Work out the finished part from the listing and answer in its coordinate system (mm). Face numbers are marked on the shaded views. A direction names the side the tool comes from. Round coordinates to 2 decimals unless told otherwise and drop trailing zeros. Order: outer loops, then holes, each group sorted by start corner. A loop starts at its lowest first (then second) coordinate and runs counter-clockwise, first axis right, second up.
Autodesk Inventor part; units mm, degrees
ref_plane "YZ Plane" through (0, 0, 0) normal (1, 0, 0) x (0, 1, 0)
ref_plane "XZ Plane" through (0, 0, 0) normal (0, 1, 0) x (-1, 0, 0)
ref_plane "XY Plane" through (0, 0, 0) normal (0, 0, 1) x (1, 0, 0)
sketch "Skizze1" plane through (0, 0, 0) normal (0, 1, 0) x (-1, 0, 0)
  line L0 (12.5, 72.5) -> (-12.5, 72.5)
  line L1 (-12.5, 72.5) -> (-12.5, -72.5)
  line L2 (-12.5, -72.5) -> (12.5, -72.5)
  line L3 (12.5, -72.5) -> (12.5, 72.5)
  point P0 (0, 0)
  point P1 (0, 72.5)
  point P2 (-12.5, 0)
  dimension "d0" = 25
  dimension "d1" = 145
extrude "Extrusion1" add sketch "Skizze1" along normal blind 100
sketch "Skizze2" plane through (12.5, 0, 72.5) normal (1, 0, 0) x (0, 0, -1)
  line L0 (0, 0) -> (145, 0) construction
  line L1 (145, 0) -> (145, 100) construction
  line L2 (0, 100) -> (145, 100) construction
  line L3 (0, 0) -> (0, 100) construction
  line L4 (0, 100) -> (80, 100)
  line L5 (80, 100) -> (80, 40)
  line L6 (80, 40) -> (0, 40)
  line L7 (0, 40) -> (0, 100)
  point P0 (72.5, 0)
  dimension "d4" = 80
  dimension "d5" = 60
extrude "Extrusion2" cut sketch "Skizze2" against normal through all
sketch "Skizze3" plane through (12.5, 0, 72.5) normal (1, 0, 0) x (0, 0, -1)
  line L0 (80, 100) -> (80, 40) construction
  line L1 (80, 40) -> (0, 40) construction
  line L2 (0, 0) -> (0, 40) construction
  line L3 (0, 0) -> (145, 0) construction
  line L4 (145, 0) -> (145, 100) construction
  line L5 (80, 100) -> (145, 100) construction
  line L6 (0, 40) -> (80, 40)
  line L7 (80, 40) -> (80, 3)
  line L8 (80, 3) -> (0, 3)
  line L9 (0, 3) -> (0, 40)
  line L10 (80, 100) -> (145, 100)
  line L11 (145, 100) -> (145, 40)
  line L12 (145, 40) -> (80, 40)
  line L13 (80, 40) -> (80, 100)
  line L14 (145, 0) -> (83, 0)
  line L15 (83, 0) -> (83, 37)
  line L16 (83, 37) -> (145, 37)
  line L17 (145, 37) -> (145, 0)
  point P0 (72.5, 0)
  dimension "d8" = 3
  dimension "d9" = 3
  dimension "d10" = 3
extrude "Extrusion3" cut sketch "Skizze3" against normal blind 22
sketch "Skizze4" plane through (-9.5, 0, 72.5) normal (1, 0, 0) x (0, 0, -1)
  line L0 (0, 40) -> (80, 40) construction
  line L1 (0, 3) -> (0, 40) construction
  line L2 (80, 3) -> (0, 3) construction
  line L3 (80, 40) -> (80, 3) construction
  line L4 (80, 40) -> (80, 3)
  line L5 (80, 3) -> (45, 3)
  line L6 (45, 3) -> (80, 40)
  line L7 (80, 3) -> (0, 3)
  line L8 (145, 0) -> (83, 0) construction
  line L9 (145, 37) -> (145, 0) construction
  line L10 (83, 37) -> (145, 37) construction
  line L11 (83, 0) -> (83, 37) construction
  line L12 (118, 37) -> (83, 3)
  line L13 (83, 37) -> (118, 37)
  line L14 (83, 3) -> (83, 37)
  line L15 (45, 3) -> (0, 3)
  line L16 (0, 0) -> (0, 40)
  line L17 (0, 40) -> (0, 3)
  line L18 (0, 40) -> (80, 40)
  line L19 (83, 3) -> (83, 0)
  line L20 (145, 0) -> (0, 0)
  line L21 (83, 0) -> (145, 0)
  line L22 (145, 37) -> (145, 0)
  line L23 (145, 0) -> (145, 37)
  line L24 (145, 37) -> (118, 37)
  point P0 (72.5, 0)
  dimension "d13" = 35
  dimension "d14" = 35
extrude "Extrusion4" cut sketch "Skizze4" against normal through all contours L6 L7 L16 L18 | L24 L22 L20 L19 L12
sketch "Skizze5" plane through (-9.5, 0, 72.5) normal (1, 0, 0) x (0, 0, -1)
  line L0 (80, 40) -> (80, 100) construction
  line L1 (145, 40) -> (80, 40) construction
  line L2 (145, 100) -> (145, 40) construction
  line L3 (80, 100) -> (145, 100) construction
  line L4 (80, 40) -> (80, 100) construction
  line L5 (80, 70) -> (145, 70) construction
  line L6 (145, 100) -> (145, 40) construction
  line L7 (80, 100) -> (145, 100) construction
  line L8 (112.5, 100) -> (112.5, 40) construction
  line L9 (145, 40) -> (80, 40) construction
  point P0 (72.5, 0)
  point P1 (88.5, 94)
  point P2 (136.5, 94)
  point P3 (136.5, 46)
  point P4 (88.5, 46)
  dimension "d17" = 48
  dimension "d18" = 48
hole "Bohrung1" at (-9.5, 94, -16) at (-9.5, 94, -64) at (-9.5, 46, -64) at (-9.5, 46, -16) direction (-1, 0, 0) diameter 4.5 end through all
sketch "Skizze6" plane through (-9.5, 0, 72.5) normal (1, 0, 0) x (0, 0, -1)
  circle A0 centre (136.5, 46) radius 2.25
  circle A1 centre (88.5, 94) radius 2.25
  circle A2 centre (136.5, 94) radius 2.25
  circle A3 centre (88.5, 46) radius 2.25
  line L0 (80, 40) -> (80, 100)
  line L1 (145, 40) -> (80, 40)
  line L2 (145, 100) -> (145, 40)
  line L3 (80, 100) -> (145, 100)
  point P0 (72.5, 0)
  point P1 (112.5, 70)
  point P2 (80, 70)
  point P3 (112.5, 100)
hole "Bohrung2" at (-9.5, 70, -40) direction (-1, 0, 0) diameter 40 end through all
sketch "Skizze7" plane through (12.5, 3, 72.5) normal (0, 1, 0) x (1, 0, 0)
  line L0 (0, 80) -> (0, 0) construction
  line L1 (0, 80) -> (-22, 80) construction
  line L2 (-22, 80) -> (-22, 45) construction
  line L3 (-22, 45) -> (-25, 45) construction
  line L4 (-25, 0) -> (-25, 45) construction
  line L5 (0, 0) -> (-25, 0) construction
  line L6 (-9.5, 13) -> (-9.5, 29)
  arc A0 (-9.5, 29) -> (-15.5, 29) centre (-12.5, 29) ccw
  line L7 (-15.5, 29) -> (-15.5, 13)
  arc A1 (-15.5, 13) -> (-9.5, 13) centre (-12.5, 13) ccw
  line L8 (-9.5, 53) -> (-9.5, 69)
  arc A2 (-9.5, 69) -> (-15.5, 69) centre (-12.5, 69) ccw
  line L9 (-15.5, 69) -> (-15.5, 53)
  arc A3 (-15.5, 53) -> (-9.5, 53) centre (-12.5, 53) ccw
  line L10 (0, 10) -> (-25, 10) construction
  line L11 (0, 32) -> (-25, 32) construction
  line L12 (0, 80) -> (0, 0) construction
  line L13 (-25, 0) -> (-25, 45) construction
  line L14 (0, 50) -> (-22, 50) construction
  line L15 (0, 72) -> (-22, 72) construction
  point P0 (-12.5, 72.5)
  point P1 (-12.5, 0)
  dimension "d33" = 6
  dimension "d34" = 22
  dimension "d35" = 10
  dimension "d36" = 40
  dimension "d37" = 22
extrude "Extrusion5" cut sketch "Skizze7" against normal through all
fillet "Rundung1" radius 2.5 4 edges at (1.5, 40, -7.5) (1.5, 37, -10.5) (0, 0, -10.5) (1.5, 3, -7.5)
equation "\"d14\" = d13"
equation "\"d37\" = d34"
properties part number "Motorhalterung_Links"
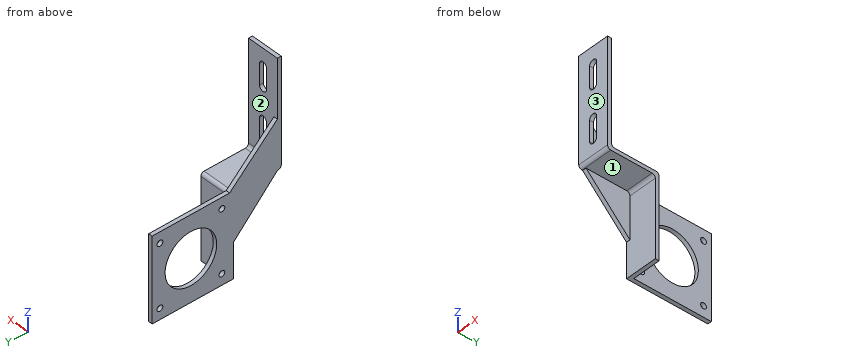
Item 1: Find section D-D (x = -6.5). Write down the section's boundary in (y, z).
Item 2: Find section A-A (z = 55). Write down the section's boundary in (x, y).
Item 3: A tool of negligible diameter and unlimited length cuts with its end or side. For the marked faces 1, 2 and 3, from which of +Z, -Z, +X, -X, +Y, -Y can it reach the whole face along a straight path? Write none if from no direction.
Item 4: Given pin 1 (10 mm diameter, centred on y = 15, z = -35.5, fed in from +X); pin 2 (11 mm diameter, centred on x = 0.5, y = 19.5, fed in from +Z); pin 3 (12.5 mm diameter, centred on x = 5.5, y = 16, fed in from -Z); pin 4 (12.5 mm diameter, centred on x = 2, z = 28, fed in from +Y), each flat-ended and moving along its own axis, determine where each tip first touches the part or whether it passes through.
Item 5: Find the intervals of material crossed by line 1 along Z through (x, y) = (-10.7, 46); line 2 along Y through (x, z) = (-11.4, -64); line 3 along Y through (x, z) = (-5.25, 59.5), in increasing order.
Item 6: Find section C-C (x = 0). Write down the section's boundary in (y, z), plus the area to 3 significant figures.
Item 7: Find section B-B (y = 94). Write down the section's boundary in (x, z).
Model answer:
1. outline: (0, -8) arc R2.5 ccw to (2.5, -10.5) - (34.5, -10.5) arc R2.5 cw to (37, -13) - (37, -72.5) - (40, -72.5) - (40, -10) arc R2.5 ccw to (37.5, -7.5) - (5.5, -7.5) arc R2.5 cw to (3, -5) - (3, 72.5) - (0, 72.5) - close
2. outline: (-12.5, 0) - (-3, 0) - (-3, 3) - (-12.5, 3) - close; (3, 0) - (12.5, 0) - (12.5, 3) - (3, 3) - close
3. face 1: -Z, +X, -Y
3. face 2: +Z, +X, +Y
3. face 3: +Z, -Z, +X, -X, -Y
4. pin 1: passes through
4. pin 2: stops at z = -7.5
4. pin 3: stops at z = -10.5
4. pin 4: stops at y = 3
5. line 1: z = -72.5 to -66.25, -61.75 to -18.25, -13.75 to -7.5
5. line 2: y = 37 to 43.75, 48.25 to 91.75, 96.25 to 100
5. line 3: y = 0 to 3
6. outline: (0, -8) arc R2.5 ccw to (2.5, -10.5) - (34.5, -10.5) arc R2.5 cw to (37, -13) - (37, -72.5) - (40, -72.5) - (40, -10) arc R2.5 ccw to (37.5, -7.5) - (5.5, -7.5) arc R2.5 cw to (3, -5) - (3, 0.5) - (0, 0.5) - close; (0, 22.5) - (3, 22.5) - (3, 40.5) - (0, 40.5) - close; (0, 62.5) - (3, 62.5) - (3, 72.5) - (0, 72.5) - close
6. area: 414 mm2
7. outline: (-12.5, -72.5) - (-9.5, -72.5) - (-9.5, -66.25) - (-12.5, -66.25) - close; (-12.5, -61.75) - (-9.5, -61.75) - (-9.5, -18.25) - (-12.5, -18.25) - close; (-12.5, -13.75) - (-9.5, -13.75) - (-9.5, -7.5) - (-12.5, -7.5) - close
